Autodesk Inventor part; units mm, degrees
ref_plane "YZ Plane" through (0, 0, 0) normal (1, 0, 0) x (0, 1, 0)
ref_plane "XZ Plane" through (0, 0, 0) normal (0, 1, 0) x (-1, 0, 0)
ref_plane "XY Plane" through (0, 0, 0) normal (0, 0, 1) x (1, 0, 0)
sketch "Sketch1" plane through (0, 0, 0) normal (0, 1, 0) x (-1, 0, 0)
  line L0 (0, 0) -> (0, 167) construction
  line L1 (0, 167) -> (-167, 167) construction
  line L2 (91.9, 0) -> (80, 0)
  line L3 (80, 0) -> (80, 86)
  line L4 (80, 86) -> (91.9, 86)
  line L5 (91.9, 86) -> (91.9, 0)
  line L6 (0, 0) -> (80, 0) construction
  line L7 (80, 86) -> (0, 86) construction
  line L8 (-167, 167) -> (-167, 247) construction
  line L9 (-167, 247) -> (-81, 247)
  line L10 (-81, 247) -> (-81, 258.9)
  line L11 (-81, 258.9) -> (-167, 258.9)
  line L12 (-167, 258.9) -> (-167, 247)
  line L13 (-81, 247) -> (-81, 167) construction
  dimension "d0" = 86
  dimension "d1" = 81
  dimension "d2" = 160
  dimension "d3" = 11.9
  dimension "d4" = 86
  dimension "d5" = 11.9
  dimension "d6" = 160
  dimension "d7" = 81
revolve "Revolution1" add sketch "Sketch1" angle 360 about axis through (0, 0, 167) along (1, 0, 0) contours L12 L11 L10 L9
revolve "Revolution2" add sketch "Sketch1" angle 360 about axis through (0, 0, 0) along (0, 0, 1) contours L2 L3 L4 L5
sketch "Sketch2" plane through (0, 0, 86) normal (0, 0, 1) x (1, 0, 0)
  line L0 (81, 43.412095) -> (81, -43.412095)
  line L1 (81, -43.412095) -> (81, 43.412095)
  line L2 (81, 80) -> (81, -80)
  line L3 (80.99, -43.430748) -> (80.99, 43.430748)
  arc A0 (81, 43.412095) -> (81, -43.412095) centre (0, 0) ccw
  circle A1 centre (0, 0) radius 91.9
  circle A2 centre (0, 0) radius 76
  dimension "d8" = 0.01
  dimension "d9" = 183.8
  dimension "d10" = 152
sketch "Sketch2 outline for Revolution3" plane through (0, 0, 86) normal (0, 0, 1) x (1, 0, 0)
  arc A0 (80.99, 43.430748) -> (80.99, -43.430748) centre (0, 0) ccw
  line L0 (80.99, -43.430748) -> (80.99, 43.430748)
  circle A1 centre (0, 0) radius 76
revolve "Revolution3" add sketch "Sketch2 outline for Revolution3" angle 90 about axis through (80.99, -43.430748, 86) along (0, 1, 0)
equation "\"d0\" = t1"
equation "\"d1\" = z1"
equation "\"d2\" = dd1"
equation "\"d3\" = s1"
equation "\"d4\" = t1"
equation "\"d5\" = s1"
equation "\"d6\" = dd1"
equation "\"d7\" = z1"
equation "\"d9\" = dd1 + 2 * s1"
equation "\"d10\" = 0.95 * dd1"
equation "\"z1\" = 81"
equation "\"t1\" = 86"
equation "\"s1\" = 11.9"
equation "\"dd1\" = 160"
properties part number "DIN 8063 Колено 90 градусов, тип W1 160" material "ПВХ, непластифицированный"
CAD build for the part. Positions are in the model's coordinates, mm. A direction names the side the tool comes from. Round coordinates to 2 decimals unless told otherwise and drop trailing zeros. Order: outer loops, then holes, each group sorted by start corner. A loop starts at its lowest first (then second) coordinate and runs counter-clockwise, first axis right, second up. Notation, with made-up numbers: (44, -37.5) - (82, -37.5) arc R27 cw to (82, -18.5) - close; hole circle Ø7 at (-0.75, -2). An arc over 180 degrees is marked (long way). Use CSV: the item, a comma, the result in double quotes. Start each with the question number.
1) Saw through at B-B (x = 113). List the corners of the cut face in (y, z), and give its area (3 significant figures).
2) Pin check, flat tips, straight feed: pin 1 Ø1 at (x, y) = (-5, 47.5) entering from +Z; pin 2 Ø8 at (x, z) = (23.5, 30.5) entering from -Y; pin 3 Ø5 at (x, z) = (114, 132) entering from +Y. Stop position of each tip, or through.
3) Tool access for faces 4 (the cylindrical face through (123.398, 24.03, 243.306)), 5 (the flat face through (167, -75.3, 139.3)), 6 (the flat face through (71, -29, 86)): list every direction of +Z, -Z, +X, -X, +Y, -Y with a clear straight run to the whole face (end or side of a thin tool).
4) Wall check: L1, parallel to Y at x = 129, z = 167; L2, parallel to Z at x = 118, y = 0. Give the ranges that are in metal, low to high. Write a range as [from, to].
5) Saw through at A-A (z = 167). Count the separate pieces of the cut face and the enclosed holes in it, and give its area (3 significant figures).
6) Two-plate mould, pull along Z, no slides. Class faces 1 (the flat face through (27.7, -75.3, 0)), 2 (the flat face through (80.99, 0.4, 243.3)), 3 (the cylindrical face through (124.602, -27.604, 254.656)): pulls with the +Z half, pulls with the -Z half, needs draft (parallel to the pull), parting line crosses it, or undercut.
7) Saw through at D-D (z = 63). List the corners of the cut face in (x, y), and give its area (3 significant figures).
Values follow:
1,outline,"circle Ø183.8 at (0, 167); hole circle Ø160 at (0, 167)"
1,area,"6,430 mm2"
2,pin 1,"stops at z = 221.01"
2,pin 2,"stops at y = -89.81"
2,pin 3,"stops at y = 85.96"
3,face 4,"+X"
3,face 5,"+Z, -Z, +X, +Y, -Y"
3,face 6,"-Z"
4,L1,"y = [-91.9, -80], [80, 91.9]"
4,L2,"z = [75.1, 87], [247, 258.9]"
5,separate pieces,"3"
5,enclosed holes,"0"
5,area,"8,420 mm2"
6,face 1,"pulls with the -Z half"
6,face 2,"undercut"
6,face 3,"parting line crosses it"
7,outline,"circle Ø183.8 at (0, 0); hole circle Ø160 at (0, 0)"
7,area,"6,430 mm2"
